Read the model definition and answer for the solid it produces. Units are mm, in the model's axes. Face numbers are marked on the shaded views. A direction names the side the tool comes from. Coordinates: 2 decimals unless noted, no trailing zeros. Order: outer loops, then holes, each group sorted by start corner. A loop starts at its lowest first (then second) coordinate and runs counter-clockwise, first axis right, second up. Notation, with made-up numbers: M 80,57 L 89,57 A18 cw 89,73 Z; hole C -20.5,36.25 d10. An arc over 180 degrees is marked long. Put each result on its own line as item: value.
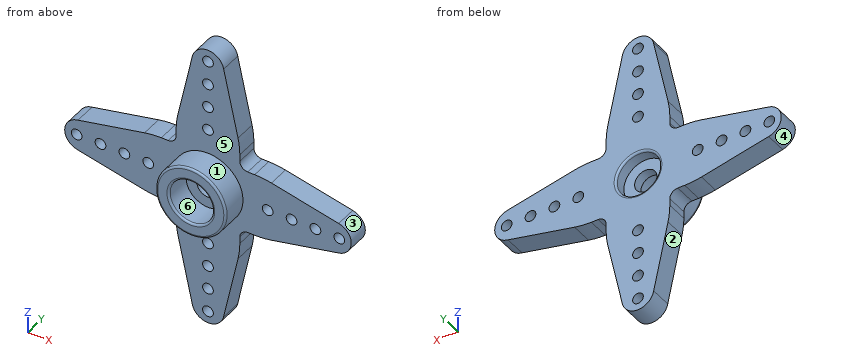
from build123d import *

# Parameters (mm, degrees)
ESQUISSE1_R             = 1.4
ESQUISSE1_R_2           = 0.675
BOSS_EXTRU_1_DEPTH      = 2.7
ESQUISSE2_R             = 2.75
ENL_V_MAT_EXTRU_1_DEPTH = 1.5
ESQUISSE3_R             = 4.4
ESQUISSE3_R_2           = 2.75
BOSS_EXTRU_2_DEPTH      = 3.3
CONG_1_R                = 0.25


with BuildPart() as part:
    # Esquisse1 → Boss.-Extru.1 (new body)
    with BuildSketch(Plane(origin=(0, 0, 0), x_dir=(1, 0, 0), z_dir=(0, 1, 0))):
        with BuildLine():
            Line((-4, 5.86229381), (-4, 5))
            ThreePointArc((-4, 5), (-4.292893219, 4.292893219), (-5, 4))
            Line((-5, 4), (-5.863381493, 4))
            ThreePointArc((-5.863381493, 4), (-6.922217369, 3.943785325), (-7.969148823, 3.775773317))
            Line((-7.969148823, 3.775773317), (-16.421153466, 1.955154663))
            ThreePointArc((-16.421153466, 1.955154663), (-17.999482643, -0.04548802), (-16.331804641, -1.972284381))
            Line((-16.331804641, -1.972284381), (-7.970163814, -3.77532015))
            ThreePointArc((-7.970163814, -3.77532015), (-6.922199111, -3.943671392), (-5.86229381, -4))
            Line((-5.86229381, -4), (-5, -4))
            ThreePointArc((-5, -4), (-4.292893219, -4.292893219), (-4, -5))
            Line((-4, -5), (-4, -5.863381493))
            ThreePointArc((-4, -5.863381493), (-3.943785325, -6.922217369), (-3.775773317, -7.969148823))
            Line((-3.775773317, -7.969148823), (-1.955154663, -16.421153466))
            ThreePointArc((-1.955154663, -16.421153466), (0.04548802, -17.999482643), (1.972284381, -16.331804641))
            Line((1.972284381, -16.331804641), (3.77532015, -7.970163814))
            ThreePointArc((3.77532015, -7.970163814), (3.943671392, -6.922199111), (4, -5.86229381))
            Line((4, -5.86229381), (4, -5))
            ThreePointArc((4, -5), (4.292893219, -4.292893219), (5, -4))
            Line((5, -4), (5.863381493, -4))
            ThreePointArc((5.863381493, -4), (6.922217369, -3.943785325), (7.969148823, -3.775773317))
            Line((7.969148823, -3.775773317), (16.421153466, -1.955154663))
            ThreePointArc((16.421153466, -1.955154663), (17.999482643, 0.04548802), (16.331804641, 1.972284381))
            Line((16.331804641, 1.972284381), (7.970163814, 3.77532015))
            ThreePointArc((7.970163814, 3.77532015), (6.922199111, 3.943671392), (5.86229381, 4))
            Line((5.86229381, 4), (5, 4))
            ThreePointArc((5, 4), (4.292893219, 4.292893219), (4, 5))
            Line((4, 5), (4, 5.863381493))
            ThreePointArc((4, 5.863381493), (3.943785325, 6.922217369), (3.775773317, 7.969148823))
            Line((3.775773317, 7.969148823), (1.955154663, 16.421153466))
            ThreePointArc((1.955154663, 16.421153466), (-0.04548802, 17.999482643), (-1.972284381, 16.331804641))
            Line((-1.972284381, 16.331804641), (-3.77532015, 7.970163814))
            ThreePointArc((-3.77532015, 7.970163814), (-3.943671392, 6.922199111), (-4, 5.86229381))
        make_face()
        Circle(ESQUISSE1_R, mode=Mode.SUBTRACT)
        with Locations((0, 16.5)):
            Circle(ESQUISSE1_R_2, mode=Mode.SUBTRACT)
        with Locations((0, 10.5)):
            Circle(ESQUISSE1_R_2, mode=Mode.SUBTRACT)
        with Locations((0, 7.5)):
            Circle(ESQUISSE1_R_2, mode=Mode.SUBTRACT)
        with Locations((0, 13.5)):
            Circle(ESQUISSE1_R_2, mode=Mode.SUBTRACT)
        with Locations((16.5, 0)):
            Circle(ESQUISSE1_R_2, mode=Mode.SUBTRACT)
        with Locations((13.5, 0)):
            Circle(ESQUISSE1_R_2, mode=Mode.SUBTRACT)
        with Locations((10.5, 0)):
            Circle(ESQUISSE1_R_2, mode=Mode.SUBTRACT)
        with Locations((7.5, 0)):
            Circle(ESQUISSE1_R_2, mode=Mode.SUBTRACT)
        with Locations((0, -16.5)):
            Circle(ESQUISSE1_R_2, mode=Mode.SUBTRACT)
        with Locations((0, -13.5)):
            Circle(ESQUISSE1_R_2, mode=Mode.SUBTRACT)
        with Locations((0, -10.5)):
            Circle(ESQUISSE1_R_2, mode=Mode.SUBTRACT)
        with Locations((0, -7.5)):
            Circle(ESQUISSE1_R_2, mode=Mode.SUBTRACT)
        with Locations((-16.5, 0)):
            Circle(ESQUISSE1_R_2, mode=Mode.SUBTRACT)
        with Locations((-13.5, 0)):
            Circle(ESQUISSE1_R_2, mode=Mode.SUBTRACT)
        with Locations((-10.5, 0)):
            Circle(ESQUISSE1_R_2, mode=Mode.SUBTRACT)
        with Locations((-7.5, 0)):
            Circle(ESQUISSE1_R_2, mode=Mode.SUBTRACT)
    extrude(amount=BOSS_EXTRU_1_DEPTH)

    # Esquisse2 → Enlèv. mat.-Extru.1 (cut)
    with BuildSketch(Plane(origin=(0, 2.7, 0), x_dir=(1, 0, 0), z_dir=(0, 1, 0))):
        Circle(ESQUISSE2_R)
    extrude(amount=-ENL_V_MAT_EXTRU_1_DEPTH, mode=Mode.SUBTRACT)

    # Esquisse3 → Boss.-Extru.2 (add)
    with BuildSketch(Plane.XZ):
        Circle(ESQUISSE3_R)
        Circle(ESQUISSE3_R_2, mode=Mode.SUBTRACT)
    extrude(amount=BOSS_EXTRU_2_DEPTH)

    # Congé1
    cong_1_edges = [part.edges().sort_by_distance(p)[0] for p in [
        (-2.75, 2.7, 0),
        (-4.4, -3.3, 0),
        (-2.75, -3.3, 0),
    ]]
    fillet(cong_1_edges, radius=CONG_1_R)


solid = part.part
Q1. Find section A-A on x = -10.5. Write down the section's boundary in (y, z) (3 decimals).
Answers below:
outline: M 0,-3.231 L 2.7,-3.231 L 2.7,-0.675 L 0,-0.675 Z; M 0,0.675 L 2.7,0.675 L 2.7,3.23 L 0,3.23 Z
Q2. A tool of negligible diameter and unlimited length cuts with its end or side. For the marked faces 1 and 2, from which of +Z, -Z, +X, -X, +Y, -Y can it reach the whole face along a straight path? Write none if from no direction.
Answers below:
face 1: -Y
face 2: -Z, -X, +Y, -Y
Q3. Find section B-B on y = -0.5. Write down the section's boundary in (x, z), plus the area to 3 significant figures.
Answers below:
outline: C 0,0 d8.8; hole C 0,0 d5.5
area: 37.1 mm^2
Q4. For a pull along X with two mould halves and no side action, classify the marked faces 3, 4, 5 and 6 as +X half, -X half, draft (parallel to the pull), parting line (faces both ways), or undercut.
Answers below:
face 3: +X half
face 4: -X half
face 5: draft
face 6: undercut
Q5. Find section C-C on z = 0. Give the number of separate pieces and of enclosed holes in the cut face, plus the area to 3 significant figures.
Answers below:
separate pieces: 10
enclosed holes: 0
area: 67.2 mm^2
Q6. Consider line 1 along Y through (x, z) = (-1, -14.5); line 2 along Z through (x, y) = (13.5, 1.9) (3 decimals); line 3 along Z through (x, y) = (-7.5, 1.3) (3 decimals). Determine where each line is inside the solid, lowest interval first.
Answers below:
line 1: y = 0 to 2.7
line 2: z = -2.583 to -0.675, 0.675 to 2.584
line 3: z = -3.865 to -0.675, 0.675 to 3.865
Q7. Given pin 1 (1.1 mm diameter, centred on x = 0, z = -10.5, fed in from +Y); pin 2 (1.5 mm diameter, centred on x = 9, y = -0.5, fed in from +Z); pin 3 (1.6 mm diameter, centred on x = 0, z = -13.5, fed in from -Y); pin 4 (2 mm diameter, centred on x = -2.5, y = 0, fed in from -Z), each flat-ended and moving along its own axis, determine where each tip first touches the part or whether it passes through.
Answers below:
pin 1: passes through
pin 2: stops at z = 3.67
pin 3: stops at y = 0
pin 4: stops at z = -17.32
